Can you work these out from the model? Positions are in its coordinate system, mm. A direction names the side the tool comes from. Give positions to 0.01 mm unless a question says otherwise; leave off trailing zeros. Order: outer loops, then holes, each group sorted by start corner. A loop starts at its lowest first (then second) coordinate and runs counter-clockwise, first axis right, second up. Notation, with made-up numbers: M 33,78.5 L 45,78.5 A31 ccw 45,108.5 Z; hole C 72,-35 d1. An arc over 180 degrees is marked long. Write each question's results on one line, items separated by ' | '.
from build123d import *

# Parameters (mm, degrees)
ESQUISSE2_R             = 1.5
ENL_V_MAT_EXTRU_1_DEPTH = 10
ESQUISSE3_R             = 8
ENL_V_MAT_EXTRU_2_DEPTH = 25
ESQUISSE4_R             = 1
ENL_V_MAT_EXTRU_3_DEPTH = 25


with BuildPart() as part:
    # Esquisse1 → Révolution1 (revolve)
    with BuildSketch(Plane.XY):
        Polygon((8, 0), (8, 1.5), (14, 1.5), (14, 30.5), (8, 30.5), (8, 32), (3, 32), (3, 0), align=None)
    revolve(axis=Axis((0, 0, 0), (0, 1, 0)))

    # Esquisse2 → Enlèv. mat.-Extru.1 (cut)
    with BuildSketch(Plane(origin=(0, 30.5, 0), x_dir=(1, 0, 0), z_dir=(0, 1, 0))):
        with Locations(Location((0, 11, 0), (0, 0, 180))):
            Circle(ESQUISSE2_R)
        with Locations(Location((9.526279442, -5.5, 0), (0, 0, 180))):
            Circle(ESQUISSE2_R)
        with Locations(Location((-9.526279442, -5.5, 0), (0, 0, 180))):
            Circle(ESQUISSE2_R)
    extrude(amount=-ENL_V_MAT_EXTRU_1_DEPTH, mode=Mode.SUBTRACT)

    # Esquisse3 → Enlèv. mat.-Extru.2 (cut)
    with BuildSketch(Plane(origin=(0, 32, 0), x_dir=(1, 0, 0), z_dir=(0, 1, 0))):
        Circle(ESQUISSE3_R)
    extrude(amount=-ENL_V_MAT_EXTRU_2_DEPTH, mode=Mode.SUBTRACT)

    # Esquisse4 → Enlèv. mat.-Extru.3 (cut)
    with BuildSketch(Plane(origin=(0, 0, 0), x_dir=(0, 0, -1), z_dir=(1, 0, 0))):
        with Locations((0, 27.5)):
            Circle(ESQUISSE4_R)
    extrude(amount=-ENL_V_MAT_EXTRU_3_DEPTH, mode=Mode.SUBTRACT)


solid = part.part
(1) For faces 1 (the face through (-10, 20.5, 6)), 2 (the face through (6, 30.5, 6)), 3 (the face through (-1.73, 0.76, 7.81)), which set-ups out of +Z, -Z, +X, -X, +Y, -Y let a thin tool reach every point of the face, with its end or its side?
Data:
face 1: +Y | face 2: +Z, -Z, +X, -X, +Y | face 3: -Y
(2) Imagine slicing it at D-D, the plane x = -8.5. Write out the boundary of the cut face in (y, z).
Data:
outline: M 1.5,-11.12 L 30.5,-11.12 L 30.5,4.41 L 20.5,4.41 L 20.5,6.59 L 30.5,6.59 L 30.5,11.12 L 1.5,11.12 Z; hole C 27.5,0 d2
(3) I need wall thicknesses on L1, parallel to Z at x = 0, y = 2.5; L2, parallel to Y at x = 8.75, z = -5. Which ranges of each line are inside material? Lowest first, please. Write a range as from..to.
Data:
L1: z = -14..-3, 3..14 | L2: y = 1.5..30.5
(4) We'd pull the mould along Y, two halves only. Please class faces 4 (the face through (-10.93, 28.49, 0.13)), 5 (the face through (11.025, 25.57, 5.566)), 6 (the face through (10, 20.5, 6)): +Y half, -Y half, draft (parallel to the pull), parting line (faces both ways), or undercut.
Data:
face 4: undercut | face 5: draft | face 6: +Y half
(5) Imagine slicing it at C-C, the plane y = 25. Write out the boundary of the cut face in (x, z), plus the area to 3 significant figures.
Data:
outline: C 0,0 d28; hole C -9.53,5.5 d3; hole C 0,0 d16; hole C 0,-11 d3; hole C 9.53,5.5 d3 | area: 393 mm2
(6) Will these pins go through, and if not, where does the flat tip stop? P1, Ø1, axis at x = -8.5, z = 9, coming from the -Y side; P2, Ø1.5, axis at x = -10, z = 6, coming from the +Y side; P3, Ø4, axis at y = 22, z = -5.5, coming from the -X side.
Data:
P1: stops at y = 1.5 | P2: stops at y = 20.5 | P3: stops at x = -13.56
(7) Imagine slicing it at B-B, the plane z = 0. Write out the boundary of the cut face in (x, y).
Data:
outline: M -14,1.5 L -8,1.5 L -8,0 L -3,0 L -3,7 L -8,7 L -8,26.5 L -14,26.5 Z; M -14,28.5 L -8,28.5 L -8,30.5 L -14,30.5 Z; M 3,0 L 8,0 L 8,1.5 L 14,1.5 L 14,30.5 L 8,30.5 L 8,7 L 3,7 Z
(8) Imagine slicing it at A-A, the plane x = 0. Write out the boundary of the cut face in (y, z).
Data:
outline: M 0,-8 L 1.5,-8 L 1.5,-14 L 30.5,-14 L 30.5,-12.5 L 20.5,-12.5 L 20.5,-9.5 L 30.5,-9.5 L 30.5,-8 L 7,-8 L 7,-3 L 0,-3 Z; M 0,3 L 7,3 L 7,8 L 30.5,8 L 30.5,14 L 1.5,14 L 1.5,8 L 0,8 Z
